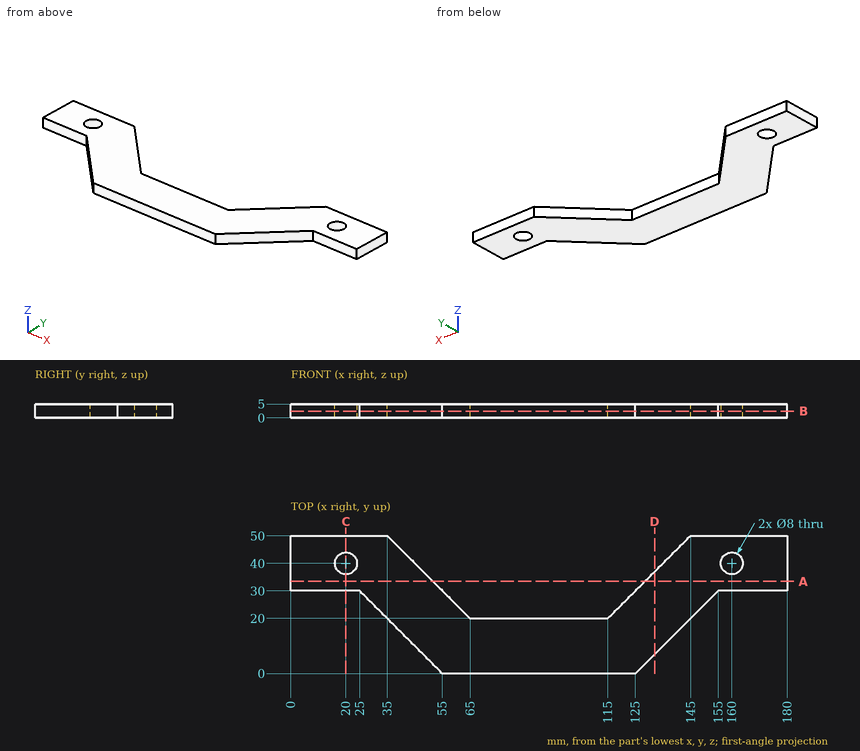
The figure shows three views and two pictorial views of one solid part (mm, origin at its lowest corner). Answer the questions. Coordinates: 2 decimals unless noted, no trailing zeros. Loops run counter-clockwise (first coordinate to the right, second up) from the corner with the lowest first, then second, coordinate; pieces in that order, holes last. Notation, with made-up numbers: (23.5, -22.75) -> (58.5, -22.75) arc R33 cw to (58.5, 8.25) -> close; hole circle Ø9 at (65, 30). An arc over 180 degrees is marked (long way). Return JSON: item names as keys, results as strings. Group by question number.
(1) A cutting plane is placed at C-C on x = 20. Write down the section's boundary in (y, z), and give its area (3 significant figures).
(2) A cutting plane is placed at B-B on z = 2.4. Write down the section's boundary in (x, y).
(3) A cutting plane is placed at A-A on y = 33.5. Write down the section's boundary in (x, z).
(4) A cutting plane is placed at D-D on x = 132. Write down the section's boundary in (y, z), and give its area (3 significant figures).
(5) Find the intervals of material crossed by probe 1 along Y at (x, z) = (160, 1.15); probe 2 along X at (y, z) = (39.5, 0.45); probe 3 along X at (y, z) = (46.5, 2.15), in increasing order. Write a range as from..to.
(6) Given pin 1 Ø1.5 at (x, z) = (164, 1.5) entering from -Y; pin 2 Ø6.5 at (x, y) = (160, 40) entering from +Z; pin 3 Ø2.5 at (x, z) = (83.5, 1.5) entering from +Y; pin 4 Ø2 at (y, z) = (28, 1) entering from -X, each flat-ended and moving along its own axis, determine where each tip first touches the part or whether it passes through.
The answers:
{
 "1": {"outline": "(30, 0) -> (36, 0) -> (36, 5) -> (30, 5) -> close; (44, 0) -> (50, 0) -> (50, 5) -> (44, 5) -> close", "area": "60.0 mm^2"},
 "2": {"outline": "(0, 30) -> (25, 30) -> (55, 0) -> (125, 0) -> (155, 30) -> (180, 30) -> (180, 50) -> (145, 50) -> (115, 20) -> (65, 20) -> (35, 50) -> (0, 50) -> close; hole circle Ø8 at (20, 40); hole circle Ø8 at (160, 40)"},
 "3": {"outline": "(0, 0) -> (51.5, 0) -> (51.5, 5) -> (0, 5) -> close; (128.5, 0) -> (180, 0) -> (180, 5) -> (128.5, 5) -> close"},
 "4": {"outline": "(7, 0) -> (37, 0) -> (37, 5) -> (7, 5) -> close", "area": "150 mm^2"},
 "5": {"probe 1": "y = 30..36, 44..50", "probe 2": "x = 0..16.03, 23.97..45.5, 134.5..156.03, 163.97..180", "probe 3": "x = 0..38.5, 141.5..180"},
 "6": {"pin 1": "stops at y = 30", "pin 2": "passes through", "pin 3": "stops at y = 20", "pin 4": "stops at x = 26"}
}
